```python
from build123d import *

# Parameters (mm, degrees)
F0_W     = 90
F0_H     = 90
F0_W_2   = 85
F0_H_2   = 85
F1_DEPTH = 30
F0_W_3   = 100
F0_H_3   = 100
F2_DEPTH = 1


with BuildPart() as f1:
    # F0 (on Top) → F1 (new body)
    with BuildSketch(Plane.XY):
        Rectangle(F0_W, F0_H)
        Rectangle(F0_W_2, F0_H_2, mode=Mode.SUBTRACT)
    extrude(amount=F1_DEPTH)

    # F0 (on Top) → F2 (join)
    with BuildSketch(Plane.XY):
        Rectangle(F0_W_3, F0_H_3)
        Rectangle(F0_W, F0_H, mode=Mode.SUBTRACT)
        Rectangle(F0_W_2, F0_H_2)
    extrude(amount=F2_DEPTH)


solid = f1.part
```
Build history of the part. All positions in model axes, mm. A direction names the side the tool comes from. Round coordinates to 2 decimals unless told otherwise and drop trailing zeros. Loops run counter-clockwise (first coordinate to the right, second up) from the corner with the lowest first, then second, coordinate; pieces in that order, holes last.
Item 1: Saw through at B-B (x = 0.5). List the corners of the cut face in (y, z).
Item 2: Which spindle directions (+Z, -Z, +X, -X, +Y, -Y) get a long thin tool onto all of the face, cutting with end or side? Do faces 1 (the face through (-1, -45, 15)), 2 (the face through (-45, -1, 15)), 3 (the face through (45, -1, 15)), 4 (the face through (42.5, -1, 15)). Say none if no direction does.
Item 3: Pin check, flat tips, straight feed: P1, Ø4, axis at y = -7.5, z = 18.5, coming from the +X side; P2, Ø12, axis at x = 11, z = 19, coming from the -Y side; P3, Ø8, axis at x = -19.5, y = -13, coming from the +Z side. Stop position of each tip, or through.
Item 4: Drill centre lines: line 1 along X through (y, z) = (8, 24.25); line 2 along Z through (x, y) = (-24, 32). Where is each one in solid material? Low to high.
Item 5: Saw through at A-A (z = 21.25). List the corners of the cut face in (x, y).
Worked answers:
1. outline: (-50, 0) - (50, 0) - (50, 1) - (45, 1) - (45, 30) - (42.5, 30) - (42.5, 1) - (-42.5, 1) - (-42.5, 30) - (-45, 30) - (-45, 1) - (-50, 1) - close
2. face 1: +Z, +X, -X, -Y
2. face 2: +Z, -X, +Y, -Y
2. face 3: +Z, +X, +Y, -Y
2. face 4: +Z
3. P1: stops at x = 45
3. P2: stops at y = -45
3. P3: stops at z = 1
4. line 1: x = -45 to -42.5, 42.5 to 45
4. line 2: z = 0 to 1
5. outline: (-45, -45) - (45, -45) - (45, 45) - (-45, 45) - close; hole (-42.5, -42.5) - (42.5, -42.5) - (42.5, 42.5) - (-42.5, 42.5) - close
